Geometry: see drawing. Coordinates: mm, zero at the bounding-box minimum. Coordinates: 2 decimals unless noted, no trailing zeros. Write each loop counter-clockwise with the first axis right and the second up, starting at its lowest first coordinate (ties: lowest second). Pieces come first, ordered by that corner, then holes. Notation, with made-up numbers: (86, -36) -> (125, -36) arc R22 ccw to (125, -29) -> close; hole circle Ø5 at (-11.75, 53.5). An arc over 180 degrees is marked (long way). Answer as a JSON object with one key per item and string values. Group by question number.
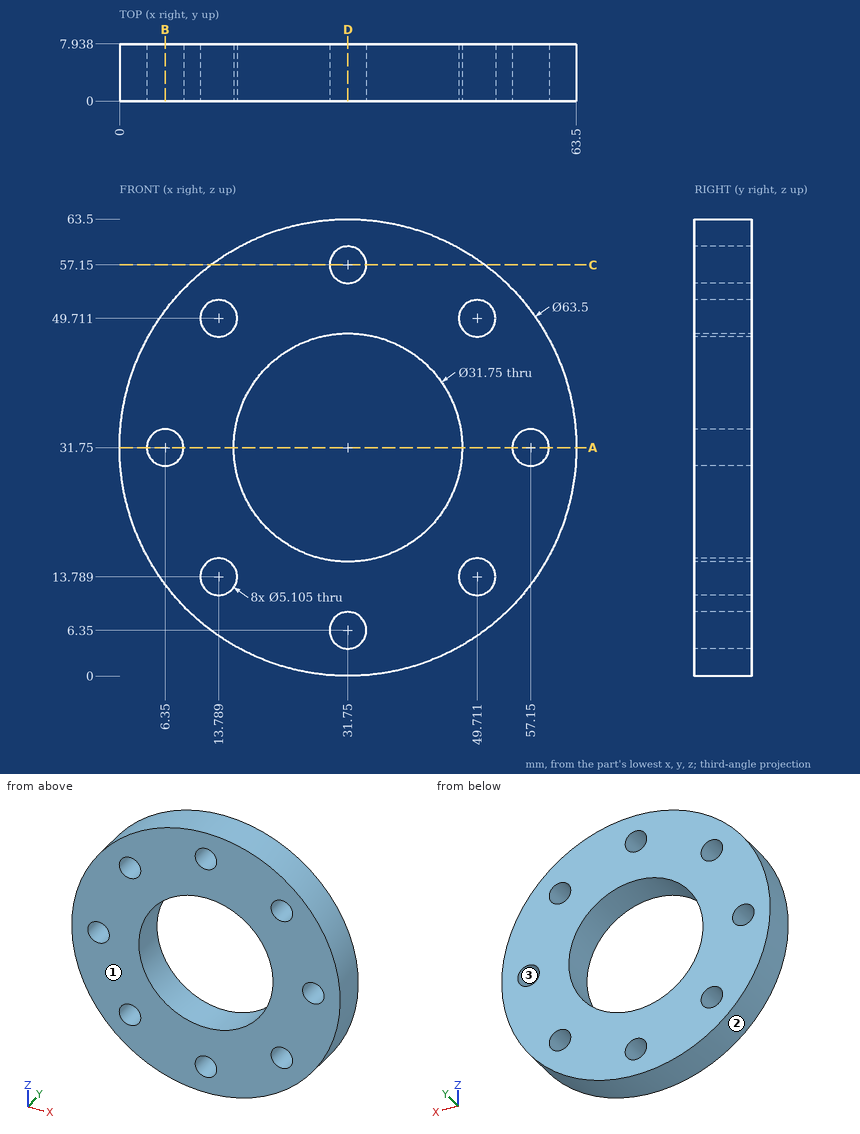
Item 1: Ray query, L1, parallel to Z at x = 32, y = 4.5; L2, parallel to X at y = 4.25, z = 12. Return the intervals inside material, ascending. Write a range as [from, to].
Item 2: Section B-B on x = 6.35. Output: boundary loops of the cut face in (y, z), then the cut area to 3 significant figures.
Item 3: Section A-A on z = 31.75. Output: boundary loops of the cut face in (x, y) (1 decimal).
Item 4: Contact query for flat-ended pins moving along their axis: pin 1 (4 mm diameter, centred on x = 22.5, y = 3, fed in from +Z); pin 2 (3 mm diameter, centred on y = 2.5, z = 23.5, fed in from +X) (1 decimal); pin 3 (3 mm diameter, centred on y = 4.5, z = 30, fed in from +X). Output: stop coordinate, or through.
Item 5: Section C-C on z = 57.15. Output: boundary loops of the cut face in (x, y), then the cut area to 3 significant figures.
Item 6: Mould query, pull axis Z, two halves, no side actions, for the marked faces 1, 2 and 3. Classes: +Z half, -Z half, draft (parallel to the pull), parting line (faces both ways), or undercut.
Item 7: Section D-D on x = 31.75. Output: boundary loops of the cut face in (y, z) (1 decimal).
Answer sheet:
{
 "1": {"L1": "z = [0, 3.81], [8.89, 15.88], [47.62, 54.61], [59.69, 63.5]", "L2": "x = [6.89, 11.97], [15.61, 47.89], [51.53, 56.61]"},
 "2": {"outline": "(0, 12.7) -> (7.94, 12.7) -> (7.94, 29.2) -> (0, 29.2) -> close; (0, 34.3) -> (7.94, 34.3) -> (7.94, 50.8) -> (0, 50.8) -> close", "area": "262 mm^2"},
 "3": {"outline": "(0, 0) -> (3.8, 0) -> (3.8, 7.9) -> (0, 7.9) -> close; (8.9, 0) -> (15.9, 0) -> (15.9, 7.9) -> (8.9, 7.9) -> close; (47.6, 0) -> (54.6, 0) -> (54.6, 7.9) -> (47.6, 7.9) -> close; (59.7, 0) -> (63.5, 0) -> (63.5, 7.9) -> (59.7, 7.9) -> close"},
 "4": {"pin 1": "stops at z = 62.66", "pin 2": "stops at x = 62.8", "pin 3": "stops at x = 63.5"},
 "5": {"outline": "(12.7, 0) -> (29.2, 0) -> (29.2, 7.94) -> (12.7, 7.94) -> close; (34.3, 0) -> (50.8, 0) -> (50.8, 7.94) -> (34.3, 7.94) -> close", "area": "262 mm^2"},
 "6": {"face 1": "draft", "face 2": "parting line", "face 3": "undercut"},
 "7": {"outline": "(0, 0) -> (7.9, 0) -> (7.9, 3.8) -> (0, 3.8) -> close; (0, 8.9) -> (7.9, 8.9) -> (7.9, 15.9) -> (0, 15.9) -> close; (0, 47.6) -> (7.9, 47.6) -> (7.9, 54.6) -> (0, 54.6) -> close; (0, 59.7) -> (7.9, 59.7) -> (7.9, 63.5) -> (0, 63.5) -> close"}
}
